from build123d import *

# Parameters (mm, degrees)
SKETCH_W         = 28.2
SKETCH_H         = 30
SKETCH_R         = 1.75
PAD_DEPTH        = 3
SKETCH002_W      = 9
SKETCH002_H      = 25
SKETCH002_W_2    = 7.9
PAD002_DEPTH     = 10
POCKET_DEPTH     = 7.25
POCKET_FACE46_W  = 25
POCKET_FACE46_H  = 7.9
PAD003_DEPTH     = 1
HOLE_D           = 2.5
HOLE_DEPTH       = 30
HOLE_CSINK_D     = 6.3
HOLE_CSINK_ANGLE = 90
CHAMFER_SIZE     = 2


with BuildPart() as inverted_body:
    # Sketch → Pad (new body)
    with BuildSketch(Plane.XY):
        with Locations((14.1, 33)):
            Rectangle(SKETCH_W, SKETCH_H)
        with Locations((10.7, 38)):
            Circle(SKETCH_R, mode=Mode.SUBTRACT)
        with Locations((25.7, 38)):
            Circle(SKETCH_R, mode=Mode.SUBTRACT)
        with Locations((25.7, 28)):
            Circle(SKETCH_R, mode=Mode.SUBTRACT)
        with Locations((10.7, 28)):
            Circle(SKETCH_R, mode=Mode.SUBTRACT)
    extrude(amount=PAD_DEPTH)

    # Sketch002 (on DatumPlane) → Pad002 (join)
    with BuildSketch(Plane.XY.offset(3)):
        with Locations((32.6, 40.5)):
            Rectangle(SKETCH002_W, SKETCH002_H)
        with Locations((3.95, 30.5)):
            Rectangle(SKETCH002_W_2, SKETCH002_H)
    extrude(amount=-PAD002_DEPTH)

    # Sketch003 → Pocket (cut)
    with BuildSketch(Plane(origin=(-0.5, 10, -7), x_dir=(1, 0, 0), z_dir=(0, 0, 1))):
        with BuildLine():
            Line((33.3, 48), (32, 48))
            Line((32, 48), (32, 18))
            Line((32, 18), (33.3, 18))
            ThreePointArc((33.3, 19), (32.8, 18.5), (33.3, 18))
            ThreePointArc((33.3, 19), (33.8, 19.5), (33.3, 20))
            ThreePointArc((33.3, 21), (32.8, 20.5), (33.3, 20))
            ThreePointArc((33.3, 21), (33.8, 21.5), (33.3, 22))
            ThreePointArc((33.3, 23), (32.8, 22.5), (33.3, 22))
            ThreePointArc((33.3, 23), (33.8, 23.5), (33.3, 24))
            ThreePointArc((33.3, 25), (32.8, 24.5), (33.3, 24))
            ThreePointArc((33.3, 25), (33.8, 25.5), (33.3, 26))
            ThreePointArc((33.3, 27), (32.8, 26.5), (33.3, 26))
            ThreePointArc((33.3, 27), (33.8, 27.5), (33.3, 28))
            ThreePointArc((33.3, 29), (32.8, 28.5), (33.3, 28))
            ThreePointArc((33.3, 29), (33.8, 29.5), (33.3, 30))
            ThreePointArc((33.3, 31), (32.8, 30.5), (33.3, 30))
            ThreePointArc((33.3, 31), (33.8, 31.5), (33.3, 32))
            ThreePointArc((33.3, 33), (32.8, 32.5), (33.3, 32))
            ThreePointArc((33.3, 33), (33.8, 33.5), (33.3, 34))
            ThreePointArc((33.3, 35), (32.8, 34.5), (33.3, 34))
            ThreePointArc((33.3, 35), (33.8, 35.5), (33.3, 36))
            ThreePointArc((33.3, 37), (32.8, 36.5), (33.3, 36))
            ThreePointArc((33.3, 37), (33.8, 37.5), (33.3, 38))
            ThreePointArc((33.3, 39), (32.8, 38.5), (33.3, 38))
            ThreePointArc((33.3, 39), (33.8, 39.5), (33.3, 40))
            ThreePointArc((33.3, 41), (32.8, 40.5), (33.3, 40))
            ThreePointArc((33.3, 41), (33.8, 41.5), (33.3, 42))
            ThreePointArc((33.3, 43), (32.8, 42.5), (33.3, 42))
            ThreePointArc((33.3, 43), (33.8, 43.5), (33.3, 44))
            ThreePointArc((33.3, 45), (32.8, 44.5), (33.3, 44))
            ThreePointArc((33.3, 45), (33.8, 45.5), (33.3, 46))
            ThreePointArc((33.3, 47), (32.8, 46.5), (33.3, 46))
            ThreePointArc((33.3, 47), (33.8, 47.5), (33.3, 48))
        make_face()
    extrude(amount=POCKET_DEPTH, mode=Mode.SUBTRACT)

    # Pocket Face46 → Pad003 (add)
    with BuildSketch(Plane(origin=(3.95, 30.5, -7), x_dir=(0, -1, 0), z_dir=(0, 0, -1))):
        Rectangle(POCKET_FACE46_W, POCKET_FACE46_H)
    extrude(amount=PAD003_DEPTH)

    # Hole
    with Locations(Plane(origin=(0, 43, 0), x_dir=(-1, 0, 0), z_dir=(0, 1, 0))):
        with Locations((-3.95, -4)):
            CounterSinkHole(HOLE_D / 2, HOLE_CSINK_D / 2, depth=HOLE_DEPTH, counter_sink_angle=HOLE_CSINK_ANGLE)

    # Chamfer
    chamfer_edges = [inverted_body.edges().sort_by_distance(p)[0] for p in [
        (28.1, 53, -2),
        (37.1, 53, -2),
        (0, 48, 1.5),
        (0, 18, -2),
        (7.9, 18, -3.5),
        (28.2, 18, 1.5),
        (37.1, 28, -2),
        (7.9, 18, -7.5),
        (0, 18, -7.5),
        (28.2, 28, 1.5),
        (28.1, 48, 1.5),
    ]]
    chamfer(chamfer_edges, length=CHAMFER_SIZE)


with BuildPart() as body:
    # Part__Mirroring: instance of inverted-body
    add(inverted_body.part.mirror(Plane(origin=(0, 0, 0), x_dir=(0, -1, 0), z_dir=(1, 0, 0))))


solid = body.part
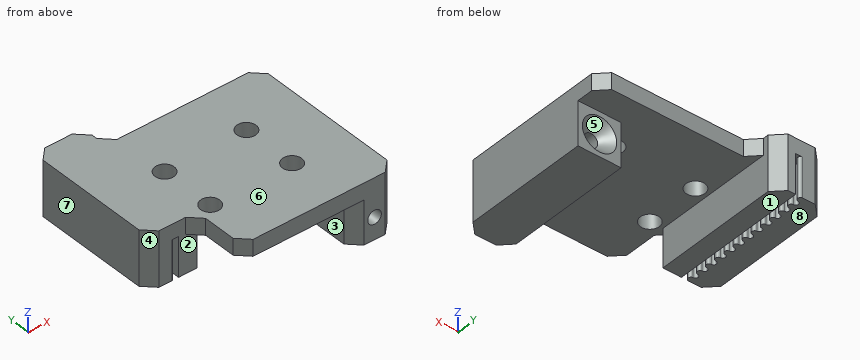
Input: part model. Units: mm. Frame: model coordinates. Face numbers are marked on the shaded views. A direction names the side the tool comes from. Round coordinates to 2 decimals unless told otherwise and drop trailing zeros. Loops run counter-clockwise (first coordinate to the right, second up) from the corner with the lowest first, then second, coordinate; pieces in that order, holes last. Notation, with made-up numbers: M -7,4 L 42,4 A13 cw 42,11 Z; hole C -36,73 d11. An arc over 180 degrees is marked long. Answer as CSV lines item,"result". Start each with the question number.
(1) Section D-D, the plane x = -22.5. Output: boundary loops of the cut face in (y, z).
(2) Section A-A, the plane y = 31.5. Output: boundary loops of the cut face in (x, z), plus the area to 3 significant figures.
(3) Section B-B, the plane y = 51.5. Output: boundary loops of the cut face in (x, z).
(4) Reachability of the marked faces 1, 2, 3 and 4 from +Z, -Z, +X, -X, +Y, -Y: full face, straight path, thin tool, end or side. Return the list, or none.
(5) First-contact query: pin 1 (1.5 mm diameter, centred on x = -20.5, y = 26, fed in from -Z); pin 2 (1.7 mm diameter, centred on x = -30, y = 37, fed in from -Z); pin 3 (2 mm diameter, centred on y = 28.5, z = -5, fed in from -X); pin 4 (6.5 mm diameter, centred on y = 27, z = -3, fed in from -X). Flat tips, straight axial feed; report the tip coordinate or a pass-through.
(6) Line query: line 1 (Y direction, x = -10.7, z = 1.1); line 2 (X direction, y = 29, z = 0.5); line 3 (X direction, y = 28.25, z = -4). Output: solid intervals per line, ascending. Write a range as [from, to].
(7) Draft query along Z for the marked faces 5, 6, 7 and 8. Return one class per face: released by +Z, released by -Z, zero draft, split by the parting line, or undercut.
(8) Section C-C, the plane z = -4. State how many separate pieces and enclosed holes the cut face has, plus the area to 3 significant figures.
Values found:
1,outline,"M 18,0 L 48,0 L 48,3 L 18,3 Z"
2,outline,"M -37.1,-7 L -33.3,-7 L -33.3,0.25 L -31.5,0.25 L -31.5,-7 L -28.1,-7 L -28.1,0 L -7.9,0 L -7.9,-8 L 0,-8 L 0,3 L -37.1,3 Z; hole C -3.95,-4 d2.5"
2,area,"220 mm²"
3,outline,"M -36.6,-7 L -33.3,-7 L -33.3,0.25 L -31.5,0.25 L -31.5,-7 L -28.6,-7 L -28.6,3 L -36.6,3 Z"
4,face 1,"-Z, -X, +Y, -Y"
4,face 2,"-Z, -X, -Y"
4,face 3,"-Z, +Y, -Y"
4,face 4,"+Z, -Z, -X, -Y"
5,pin 1,"stops at z = 0"
5,pin 2,"stops at z = -7"
5,pin 3,"stops at x = -36.6"
5,pin 4,"stops at x = -37.1"
6,line 1,"y = [18, 26.25], [29.75, 36.25], [39.75, 48]"
6,line 2,"x = [-36.1, -27.14], [-24.26, -12.14], [-9.26, 0]"
6,line 3,"x = [-35.35, -32.37], [-31.5, -28.1], [-7.9, -5.2], [-2.7, 0]"
7,face 5,"undercut"
7,face 6,"released by +Z"
7,face 7,"zero draft"
7,face 8,"released by -Z"
8,separate pieces,"4"
8,enclosed holes,"0"
8,area,"314 mm²"
